```python
from build123d import *

# Parameters (mm, degrees)
EXTRUSION1_DEPTH = 50
EXTRUSION2_REACH = 24.627
ESQUISSE3_R      = 2.5
EXTRUSION3_REACH = 39.213
ESQUISSE4_R      = 1.5


with BuildPart() as part:
    # Esquisse1 → Extrusion1 (new body)
    with BuildSketch(Plane(origin=(0, 0, 0), x_dir=(1, 0, 0), z_dir=(0, 1, 0))):
        Polygon((0, 0), (0, 30), (21.213203436, 51.213203436), (22.627416998, 49.798989873), (2, 29.171572875), (2, 0), align=None)
    extrude(amount=EXTRUSION1_DEPTH)

    # Esquisse3 → Extrusion2 (cut, up to next)
    with BuildSketch(Plane.ZY, mode=Mode.PRIVATE) as extrusion2_sk1:
        with Locations((-15, 5)):
            Circle(ESQUISSE3_R)
    extrusion2_tool1 = extrude(extrusion2_sk1.sketch, amount=-EXTRUSION2_REACH, mode=Mode.PRIVATE) & part.part
    add(extrusion2_tool1.solids().sort_by_distance((0, 5, -15))[0], mode=Mode.SUBTRACT)
    # Esquisse3 → Extrusion2 (cut, up to next)
    with BuildSketch(Plane.ZY, mode=Mode.PRIVATE) as extrusion2_sk2:
        with Locations((-15, 45)):
            Circle(ESQUISSE3_R)
    extrusion2_tool2 = extrude(extrusion2_sk2.sketch, amount=-EXTRUSION2_REACH, mode=Mode.PRIVATE) & part.part
    add(extrusion2_tool2.solids().sort_by_distance((0, 45, -15))[0], mode=Mode.SUBTRACT)

    # Esquisse4 → Extrusion3 (cut, up to next)
    with BuildSketch(Plane(origin=(-15, 0, -15), x_dir=(-0.707106781, 0, 0.707106781), z_dir=(-0.707106781, 0, -0.707106781)), mode=Mode.PRIVATE) as extrusion3_sk1:
        with Locations((-36.213203436, 43.5)):
            Circle(ESQUISSE4_R)
    extrusion3_tool1 = extrude(extrusion3_sk1.sketch, amount=-EXTRUSION3_REACH, mode=Mode.PRIVATE) & part.part
    add(extrusion3_tool1.solids().sort_by_distance((10.606602, 43.5, -40.606602))[0], mode=Mode.SUBTRACT)
    # Esquisse4 → Extrusion3 (cut, up to next)
    with BuildSketch(Plane(origin=(-15, 0, -15), x_dir=(-0.707106781, 0, 0.707106781), z_dir=(-0.707106781, 0, -0.707106781)), mode=Mode.PRIVATE) as extrusion3_sk2:
        with Locations((-36.213203436, 6.5)):
            Circle(ESQUISSE4_R)
    extrusion3_tool2 = extrude(extrusion3_sk2.sketch, amount=-EXTRUSION3_REACH, mode=Mode.PRIVATE) & part.part
    add(extrusion3_tool2.solids().sort_by_distance((10.606602, 6.5, -40.606602))[0], mode=Mode.SUBTRACT)


solid = part.part
```
The model under review builds one solid part; all positions refer to its coordinate system, in mm. A direction names the side the tool comes from. Give positions to 0.01 mm unless a question says otherwise; leave off trailing zeros. Write each loop counter-clockwise with the first axis right and the second up, starting at its lowest first coordinate (ties: lowest second). Pieces come first, ordered by that corner, then holes. Notation, with made-up numbers: M -28.5,48 L 14.5,48 A15 cw 14.5,55 Z; hole C 39.5,42 d9. An arc over 180 degrees is marked long. Write each question's results on one line, items separated by ' | '. Start each with the question number.
1. We need section A-A (z = -15). Write out the cut boundary in (x, y).
2. Mouldability with a two-part tool opening along Y and no side actions: class faces 1 (the cylindrical face through (10.81, 5.17, -39.42)), 2 (the cylindrical face through (0.99, 6.69, -16.84)), 3 (the flat face through (21.91, 24.65, -50.516)), 4 (the flat face through (3.8, 50, -31.4)) as released by +Y, released by -Y, zero draft, split by the parting line, or undercut.
3. We need section C-C (x = 7.25). Write out the cut boundary in (y, z), and give its area (3 significant figures).
4. Insertion check: pin 1 Ø8 at (x, y) = (9.5, 34) entering from -Z; pin 2 Ø9 at (y, z) = (15, -8.5) entering from +X; pin 3 Ø8 at (x, y) = (7.5, 8) entering from -Z. Each pin has a flat end and moves straight along its axis. Give the tip position at first contact, or say it passes through.
5. For probe 1 along Y at (x, z) = (1, -15); probe 2 along X at (y, z) = (34, -29); probe 3 along Z at (x, y) = (21.5, 25), list the stretches that pass through material, from the lowest coordinate up. Write a range as [from, to].
6. We need section D-D (z = -27). Write out the cut boundary in (x, y), and give its area (3 significant figures).
7. For faces 5 (the flat face through (2, 25, -15)), 6 (the flat face through (3.8, 0, -31.4)), list the 3-axis set-ups (+Z, -Z, +X, -X, +Y, -Y) from which the entire face can be reached by the end or side of a thin tool; tool diameter is ignored.
8. We need section B-B (y = 36). Write out the cut boundary in (x, z).
Results found:
1) outline: M 0,0 L 2,0 L 2,2.5 L 0,2.5 Z; M 0,7.5 L 2,7.5 L 2,42.5 L 0,42.5 Z; M 0,47.5 L 2,47.5 L 2,50 L 0,50 Z
2) face 1: undercut | face 2: undercut | face 3: zero draft | face 4: released by +Y
3) outline: M 0,-37.25 L 50,-37.25 L 50,-34.42 L 0,-34.42 Z | area: 141 mm^2
4) pin 1: stops at z = -43.5 | pin 2: stops at x = 2 | pin 3: stops at z = -41.5
5) probe 1: y = [0, 2.5], [7.5, 42.5], [47.5, 50] | probe 2: x = [0, 2] | probe 3: z = [-50.93, -48.67]
6) outline: M 0,0 L 2,0 L 2,50 L 0,50 Z | area: 100 mm^2
7) face 5: +Z, +X, +Y, -Y | face 6: +Z, -Z, +X, -X, -Y
8) outline: M 0,-30 L 21.21,-51.21 L 22.63,-49.8 L 2,-29.17 L 2,0 L 0,0 Z
